Build history of the part. All positions in model axes, mm. A direction names the side the tool comes from. Give positions to 0.01 mm unless a question says otherwise; leave off trailing zeros. Write each loop counter-clockwise with the first axis right and the second up, starting at its lowest first coordinate (ties: lowest second). Pieces come first, ordered by that corner, then holes. Notation, with made-up numbers: (61, 17.5) -> (104, 17.5) arc R18 ccw to (104, 39.5) -> close; hole circle Ø5 at (-8, 88). An arc over 180 degrees is marked (long way). Put each result on its own line as item: value. Start each with the question number.
Item 1: Flat gauge pins, fed straight in: pin 1 Ø5.5 at (y, z) = (-8.89, 12.192) entering from +X; pin 2 Ø1.4 at (y, z) = (-9.5, -11.5) entering from +X. Where does each tip first touch, or does it go through?
Item 2: Tool access for faces 5 (the cylindrical face through (1.628, -14.218, -7.255)), 6 (the cylindrical face through (2.63, 3.243, -10.297)), 7 (the flat face through (2.286, 0, 25)): list every direction of +Z, -Z, +X, -X, +Y, -Y with a clear straight run to the whole face (end or side of a thin tool).
Item 3: Slice it at B-B, the plane x = 1. List the corners of the cut face in (y, z) (1 decimal), plus the area to 3 significant figures.
Item 4: Drill centre lines: line 1 along Z through (x, y) = (2, -13.97); line 2 along Z through (x, y) = (7.5, 9); line 3 along Z through (x, y) = (13, -0.5). Where is each one in solid material? Low to high.
Item 5: Two-plate mould, pull along Y, no slides. Class faces 1 (the flat face through (4.064, -9, -12)), 2 (the cylindrical face through (7.8, 16.9, 42)), 3 (the flat face through (8, 0, -18.098)), 4 (the flat face through (3.302, 14, 33)): pulls with the +Y half, pulls with the -Y half, needs draft (parallel to the pull), parting line crosses it, or undercut.
Item 6: Slice it at D-D, the plane x = 12.75. Give the number of separate pieces and of enclosed holes in the cut face, plus the area to 3 significant figures.
```python
from build123d import *

# Parameters (mm, degrees)
SKETCH1_R             = 10.795
BOSS_EXTRUDE1_DEPTH   = 15.875
CAVITY1_START         = 5.334
CAVITY1_OUTLINE_R     = 1.143
CAVITY1_OUTLINE_R_2   = 4.445
CAVITY1_OUTLINE_R_3   = 10.795
CAVITY1_DEPTH         = 10.541
CAVITY1_START_2       = 15.494
CAVITY1_2_OUTLINE_R   = 1.143
CAVITY1_2_OUTLINE_R_2 = 4.445
CAVITY1_2_DEPTH       = 0.381
CAVITY1_START_3       = 2.286
CAVITY1_3_OUTLINE_R   = 1.143
CAVITY1_3_OUTLINE_R_2 = 4.445
CAVITY1_3_DEPTH       = 3.048
CAVITY1_4_OUTLINE_R   = 1.905
CAVITY1_4_DEPTH       = 3.302
CAVITY1_START_4       = 13.716
CAVITY1_5_DEPTH       = 1.778
CAVITY1_START_5       = 4.064
CAVITY1_6_OUTLINE_R   = 2.286
CAVITY1_6_DEPTH       = 1.27
CAVITY1_START_6       = 2.032
CAVITY1_7_DEPTH       = 0.254
CUT_EXTRUDE1_REACH    = 51.711
SKETCH2_R             = 2.286
SKETCH3_R             = 4.445
CUT_EXTRUDE2_DEPTH    = 5.969


# Read off the part's stored shape, not the designer's step: Cavity1
with BuildPart() as part:
    # Sketch1 → Boss-Extrude1 (new body)
    with BuildSketch(Plane(origin=(0, 0, 0), x_dir=(0, 0, -1), z_dir=(1, 0, 0))):
        with BuildLine():
            Line((12.954, 18.415), (-38.354, 18.415))
            ThreePointArc((-38.354, 18.415), (-41.991003729, 16.908503729), (-43.4975, 13.2715))
            Line((-43.4975, 13.2715), (-43.4975, -13.2715))
            ThreePointArc((-43.4975, -13.2715), (-41.991003729, -16.908503729), (-38.354, -18.415))
            Line((-38.354, -18.415), (12.954, -18.415))
            ThreePointArc((12.954, -18.415), (16.591003729, -16.908503729), (18.0975, -13.2715))
            Line((18.0975, -13.2715), (18.0975, 13.2715))
            ThreePointArc((18.0975, 13.2715), (16.591003729, 16.908503729), (12.954, 18.415))
        make_face()
        Circle(SKETCH1_R, mode=Mode.SUBTRACT)
    extrude(amount=BOSS_EXTRUDE1_DEPTH)

    # Cavity1 outline → Cavity1 (cut)
    # profile 1 of 6: a face of its own
    with BuildSketch(Plane.YZ.offset(CAVITY1_START)):
        with Locations((13.97, 34.544)):
            Circle(CAVITY1_OUTLINE_R)
    # profile 2 of 6: a face of its own
    with BuildSketch(Plane.YZ.offset(CAVITY1_START)):
        with Locations((0, 25.4)):
            Circle(CAVITY1_OUTLINE_R_2)
    # profile 3 of 6: a face of its own
    with BuildSketch(Plane.YZ.offset(CAVITY1_START)):
        with BuildLine():
            ThreePointArc((6.663505747, 12.710188518), (0, 14.351), (-6.663505747, 12.710188518))
            ThreePointArc((-6.663505747, 12.710188518), (-10.236847552, 14.039105214), (-10.064128852, 10.230567504))
            ThreePointArc((-10.064128852, 10.230567504), (-14.351, 0), (-10.064128852, -10.230567504))
            ThreePointArc((-10.064128852, -10.230567504), (-10.236847552, -14.039105214), (-6.663505747, -12.710188518))
            ThreePointArc((-6.663505747, -12.710188518), (0, -14.351), (6.663505747, -12.710188518))
            ThreePointArc((6.663505747, -12.710188518), (10.236847552, -14.039105214), (10.064128852, -10.230567504))
            ThreePointArc((10.064128852, -10.230567504), (14.351, 0), (10.064128852, 10.230567504))
            ThreePointArc((10.064128852, 10.230567504), (10.236847552, 14.039105214), (6.663505747, 12.710188518))
        make_face()
        Circle(CAVITY1_OUTLINE_R_3, mode=Mode.SUBTRACT)
    # profile 4 of 6: a face of its own
    with BuildSketch(Plane.YZ.offset(CAVITY1_START)):
        with Locations((13.97, -9.144)):
            Circle(CAVITY1_OUTLINE_R)
    # profile 5 of 6: a face of its own
    with BuildSketch(Plane.YZ.offset(CAVITY1_START)):
        with Locations((-13.97, 34.544)):
            Circle(CAVITY1_OUTLINE_R)
    # profile 6 of 6: a face of its own
    with BuildSketch(Plane.YZ.offset(CAVITY1_START)):
        with Locations((-13.97, -9.144)):
            Circle(CAVITY1_OUTLINE_R)
    extrude(amount=CAVITY1_DEPTH, mode=Mode.SUBTRACT)

    # Cavity1 2 outline → Cavity1 2 (cut)
    with BuildSketch(Plane.YZ.offset(CAVITY1_START_2)):
        with BuildLine():
            ThreePointArc((16.8275, 38.354), (15.785971714, 40.868471714), (13.2715, 41.91))
            Line((13.2715, 41.91), (-13.2715, 41.91))
            ThreePointArc((-13.2715, 41.91), (-15.785971714, 40.868471714), (-16.8275, 38.354))
            Line((-16.8275, 38.354), (-16.8275, -12.954))
            ThreePointArc((-16.8275, -12.954), (-15.785971714, -15.468471714), (-13.2715, -16.51))
            Line((-13.2715, -16.51), (13.2715, -16.51))
            ThreePointArc((13.2715, -16.51), (15.785971714, -15.468471714), (16.8275, -12.954))
            Line((16.8275, -12.954), (16.8275, 38.354))
        make_face()
        with Locations((13.97, 34.544)):
            Circle(CAVITY1_2_OUTLINE_R, mode=Mode.SUBTRACT)
        with BuildLine():
            ThreePointArc((10.064128852, 10.230567504), (14.351, 0), (10.064128852, -10.230567504))
            ThreePointArc((10.064128852, -10.230567504), (10.236847552, -14.039105214), (6.663505747, -12.710188518))
            ThreePointArc((6.663505747, -12.710188518), (0, -14.351), (-6.663505747, -12.710188518))
            ThreePointArc((-6.663505747, -12.710188518), (-10.236847552, -14.039105214), (-10.064128852, -10.230567504))
            ThreePointArc((-10.064128852, -10.230567504), (-14.351, 0), (-10.064128852, 10.230567504))
            ThreePointArc((-10.064128852, 10.230567504), (-10.236847552, 14.039105214), (-6.663505747, 12.710188518))
            ThreePointArc((-6.663505747, 12.710188518), (0, 14.351), (6.663505747, 12.710188518))
            ThreePointArc((6.663505747, 12.710188518), (10.236847552, 14.039105214), (10.064128852, 10.230567504))
        make_face(mode=Mode.SUBTRACT)
        with Locations((0, 25.4)):
            Circle(CAVITY1_2_OUTLINE_R_2, mode=Mode.SUBTRACT)
        with Locations((13.97, -9.144)):
            Circle(CAVITY1_2_OUTLINE_R, mode=Mode.SUBTRACT)
        with Locations((-13.97, 34.544)):
            Circle(CAVITY1_2_OUTLINE_R, mode=Mode.SUBTRACT)
        with Locations((-13.97, -9.144)):
            Circle(CAVITY1_2_OUTLINE_R, mode=Mode.SUBTRACT)
    extrude(amount=CAVITY1_2_DEPTH, mode=Mode.SUBTRACT)

    # Cavity1 3 outline → Cavity1 3 (cut)
    with BuildSketch(Plane.YZ.offset(CAVITY1_START_3)):
        with Locations((13.97, 34.544)):
            Circle(CAVITY1_3_OUTLINE_R)
        with Locations((0, 25.4)):
            Circle(CAVITY1_3_OUTLINE_R_2)
        with BuildLine():
            ThreePointArc((3.011692939, 10.366375), (3.7542861, 12.050819068), (3.62043784, 13.886815))
            ThreePointArc((3.62043784, 13.886815), (0, 14.351), (-3.62043784, 13.886815))
            ThreePointArc((-3.62043784, 13.886815), (-3.7542861, 12.050819068), (-3.011692939, 10.366375))
            ThreePointArc((-3.011692939, 10.366375), (0, 10.795), (3.011692939, 10.366375))
        make_face()
        with Locations((13.97, -9.144)):
            Circle(CAVITY1_3_OUTLINE_R)
        with Locations((-13.97, 34.544)):
            Circle(CAVITY1_3_OUTLINE_R)
        with Locations((-13.97, -9.144)):
            Circle(CAVITY1_3_OUTLINE_R)
    extrude(amount=CAVITY1_3_DEPTH, mode=Mode.SUBTRACT)

    # Cavity1 4 outline → Cavity1 4 (cut)
    with BuildSketch(Plane.YZ):
        with Locations((13.97, 34.544)):
            Circle(CAVITY1_4_OUTLINE_R)
        with Locations((13.97, -9.144)):
            Circle(CAVITY1_4_OUTLINE_R)
        with Locations((-13.97, 34.544)):
            Circle(CAVITY1_4_OUTLINE_R)
        with Locations((-13.97, -9.144)):
            Circle(CAVITY1_4_OUTLINE_R)
    extrude(amount=CAVITY1_4_DEPTH, mode=Mode.SUBTRACT)

    # Cavity1 5 outline → Cavity1 5 (cut)
    with BuildSketch(Plane.YZ.offset(CAVITY1_START_4)):
        with BuildLine():
            Line((4.32851275, 24.389058668), (6.269761763, 26.298725967))
            ThreePointArc((6.269761763, 26.298725967), (6.329908656, 26.800266009), (6.35, 27.305))
            ThreePointArc((6.35, 27.305), (5.350674614, 30.724470892), (2.667234274, 33.067669635))
            Line((2.667234274, 33.067669635), (1.522653349, 29.576068938))
            ThreePointArc((1.522653349, 29.576068938), (3.641855237, 27.948512396), (4.445, 25.4))
            ThreePointArc((4.445, 25.4), (4.41578216, 24.891184794), (4.32851275, 24.389058668))
        make_face()
        with BuildLine():
            ThreePointArc((1.261900966, 21.081648335), (4.581043617, 22.907666788), (6.269761763, 26.298725967))
            Line((6.269761763, 26.298725967), (4.32851275, 24.389058668))
            ThreePointArc((4.32851275, 24.389058668), (3.227510813, 22.343662494), (1.245086431, 21.132941906))
            Line((1.245086431, 21.132941906), (1.261900966, 21.081648335))
        make_face()
        with BuildLine():
            ThreePointArc((0.903307826, 21.019577582), (1.083049155, 21.048043509), (1.261900966, 21.081648335))
            Line((1.261900966, 21.081648335), (1.245086431, 21.132941906))
            ThreePointArc((1.245086431, 21.132941906), (1.093135949, 21.091510845), (0.939813075, 21.055488936))
            Line((0.939813075, 21.055488936), (0.903307826, 21.019577582))
        make_face()
        with BuildLine():
            ThreePointArc((3.3e-08, 20.955), (0.452806623, 20.971164972), (0.903307826, 21.019577582))
            Line((0.903307826, 21.019577582), (0.939813075, 21.055488936))
            ThreePointArc((0.939813075, 21.055488936), (0.472585099, 20.980193633), (3.3e-08, 20.955))
        make_face()
        with BuildLine():
            Line((1.522653349, 29.576068938), (2.667234274, 33.067669635))
            ThreePointArc((2.667234274, 33.067669635), (0, 33.655), (-2.667234274, 33.067669635))
            Line((-2.667234274, 33.067669635), (-1.522653349, 29.576068938))
            ThreePointArc((-1.522653349, 29.576068938), (0, 29.845), (1.522653349, 29.576068938))
        make_face()
        with BuildLine():
            ThreePointArc((-0.903307826, 21.019577582), (-0.45280659, 20.97116497), (3.3e-08, 20.955))
            ThreePointArc((3.3e-08, 20.955), (-0.472585066, 20.980193629), (-0.939813075, 21.055488936))
            Line((-0.939813075, 21.055488936), (-0.903307826, 21.019577582))
        make_face()
        with BuildLine():
            Line((-1.522653349, 29.576068938), (-2.667234274, 33.067669635))
            ThreePointArc((-2.667234274, 33.067669635), (-5.605544054, 30.288349771), (-6.269761763, 26.298725967))
            Line((-6.269761763, 26.298725967), (-4.32851275, 24.389058668))
            ThreePointArc((-4.32851275, 24.389058668), (-3.909642575, 27.514880596), (-1.522653349, 29.576068938))
        make_face()
        with BuildLine():
            ThreePointArc((-1.261900966, 21.081648335), (-1.083049155, 21.048043509), (-0.903307826, 21.019577582))
            Line((-0.903307826, 21.019577582), (-0.939813075, 21.055488936))
            ThreePointArc((-0.939813075, 21.055488936), (-1.093135949, 21.091510845), (-1.245086431, 21.132941906))
            Line((-1.245086431, 21.132941906), (-1.261900966, 21.081648335))
        make_face()
        with BuildLine():
            Line((-4.32851275, 24.389058668), (-6.269761763, 26.298725967))
            ThreePointArc((-6.269761763, 26.298725967), (-4.581043617, 22.907666788), (-1.261900966, 21.081648335))
            Line((-1.261900966, 21.081648335), (-1.245086431, 21.132941906))
            ThreePointArc((-1.245086431, 21.132941906), (-3.227510813, 22.343662494), (-4.32851275, 24.389058668))
        make_face()
    extrude(amount=CAVITY1_5_DEPTH, mode=Mode.SUBTRACT)

    # Cavity1 6 outline → Cavity1 6 (cut)
    with BuildSketch(Plane.YZ.offset(CAVITY1_START_5)):
        with Locations((8.89, 12.192)):
            Circle(CAVITY1_6_OUTLINE_R)
        with Locations((8.89, -12.192)):
            Circle(CAVITY1_6_OUTLINE_R)
        with Locations((-8.89, 12.192)):
            Circle(CAVITY1_6_OUTLINE_R)
        with Locations((-8.89, -12.192)):
            Circle(CAVITY1_6_OUTLINE_R)
    extrude(amount=CAVITY1_6_DEPTH, mode=Mode.SUBTRACT)

    # Cavity1 7 outline → Cavity1 7 (cut)
    with BuildSketch(Plane.YZ.offset(CAVITY1_START_6)):
        with BuildLine():
            ThreePointArc((3.011692939, 10.366375), (3.7542861, 12.050819068), (3.62043784, 13.886815))
            ThreePointArc((3.62043784, 13.886815), (0, 14.351), (-3.62043784, 13.886815))
            ThreePointArc((-3.62043784, 13.886815), (-3.7542861, 12.050819068), (-3.011692939, 10.366375))
            ThreePointArc((-3.011692939, 10.366375), (0, 10.795), (3.011692939, 10.366375))
        make_face()
    extrude(amount=CAVITY1_7_DEPTH, mode=Mode.SUBTRACT)

    # Sketch2 → Cut-Extrude1 (cut, up to next)
    with BuildSketch(Plane(origin=(15.494, 0, 0), x_dir=(0, 0, -1), z_dir=(1, 0, 0)), mode=Mode.PRIVATE) as cut_extrude1_sk1:
        with Locations((-25.4, 12.3825)):
            Circle(SKETCH2_R)
    cut_extrude1_tool1 = extrude(cut_extrude1_sk1.sketch, amount=-CUT_EXTRUDE1_REACH, mode=Mode.PRIVATE) & part.part
    # Sketch2 → Cut-Extrude1 (cut, up to next)
    with BuildSketch(Plane(origin=(15.494, 0, 0), x_dir=(0, 0, -1), z_dir=(1, 0, 0)), mode=Mode.PRIVATE) as cut_extrude1_sk2:
        with Locations((-25.4, -12.3825)):
            Circle(SKETCH2_R)
    cut_extrude1_tool2 = extrude(cut_extrude1_sk2.sketch, amount=-CUT_EXTRUDE1_REACH, mode=Mode.PRIVATE) & part.part
    add(cut_extrude1_tool1.solids().sort_by_distance((15.494, 12.3825, 25.4))[0], mode=Mode.SUBTRACT)
    add(cut_extrude1_tool2.solids().sort_by_distance((15.494, -12.3825, 25.4))[0], mode=Mode.SUBTRACT)

    # Sketch3 → Cut-Extrude2 (cut)
    with BuildSketch(Plane(origin=(15.494, 0, 0), x_dir=(0, 0, -1), z_dir=(1, 0, 0))):
        with Locations((-25.4, 12.3825)):
            Circle(SKETCH3_R)
        with Locations((-25.4, -12.3825)):
            Circle(SKETCH3_R)
    extrude(amount=-CUT_EXTRUDE2_DEPTH, mode=Mode.SUBTRACT)


solid = part.part
```
Values follow:
1. pin 1: x = 15.49
1. pin 2: x = 4.06
2. face 5: -X
2. face 6: +X, -X
2. face 7: +X
3. outline: (-18.4, -13) arc R5.1 ccw to (-13.3, -18.1) -> (13.3, -18.1) arc R5.1 ccw to (18.4, -13) -> (18.4, 38.4) arc R5.1 ccw to (13.3, 43.5) -> (-13.3, 43.5) arc R5.1 ccw to (-18.4, 38.4) -> close; hole circle Ø3.8 at (-14, -9.1); hole circle Ø3.8 at (-14, 34.5); hole circle Ø4.6 at (-12.4, 25.4); hole circle Ø21.6 at (0, 0); hole circle Ø4.6 at (12.4, 25.4); hole circle Ø3.8 at (14, -9.1); hole circle Ø3.8 at (14, 34.5)
3. area: 1,800 mm2
4. line 1: -18.05 to -11.05, -7.24 to 23.76, 27.04 to 32.64, 36.45 to 43.45
4. line 2: -18.1 to -14.48, 14.48 to 43.5
4. line 3: -18.1 to -14.34, 14.34 to 20.98, 29.82 to 43.5
5. face 1: undercut
5. face 2: pulls with the +Y half
5. face 3: needs draft
5. face 4: undercut
6. separate pieces: 1
6. enclosed holes: 8
6. area: 1,350 mm2
